Here's how the part is built. I have some questions about the finished solid (model axes, mm). Face numbers are marked on the shaded views. A direction names the side the tool comes from. Coordinates: 2 decimals unless noted, no trailing zeros. Loops run counter-clockwise (first coordinate to the right, second up) from the corner with the lowest first, then second, coordinate; pieces in that order, holes last.
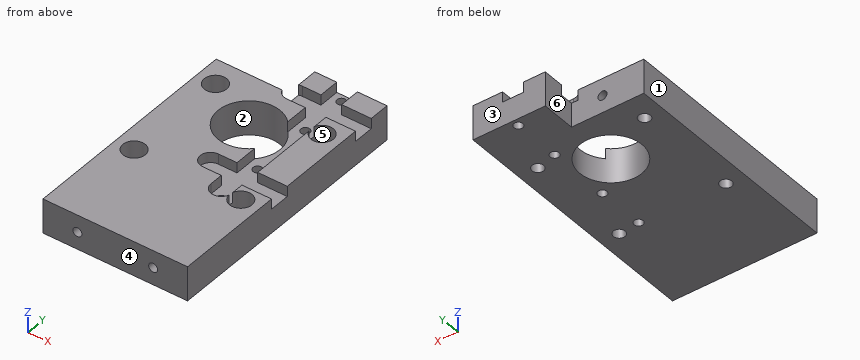
```python
from build123d import *

# Parameters (mm, degrees)
BOSS_EXTRUDE1_DEPTH                      = 10
CUT_EXTRUDE1_REACH                       = 89.407
SKETCH2_R                                = 9
CUT_EXTRUDE2_DEPTH                       = 3
CBORE_FOR_M3_PAN_HEAD_SCREW1_D           = 3.4
CBORE_FOR_M3_PAN_HEAD_SCREW1_CBORE_D     = 6.5
CBORE_FOR_M3_PAN_HEAD_SCREW1_CBORE_DEPTH = 6.5
M3X0_5_TAPPED_HOLE1_D                    = 2.6
M3X0_5_TAPPED_HOLE2_D                    = 2.6
M3X0_5_TAPPED_HOLE2_DEPTH                = 9
M3X0_5_TAPPED_HOLE2_TIP                  = 0.781118805
M3X0_5_TAPPED_HOLE3_D                    = 2.6
M3X0_5_TAPPED_HOLE3_DEPTH                = 9
M3X0_5_TAPPED_HOLE3_TIP                  = 0.781118805


with BuildPart() as part:
    # Sketch1 → Boss-Extrude1 (new body)
    with BuildSketch(Plane.XY):
        Polygon((0, 0), (42, 0), (42, 66), (42, 76), (21, 76), (21, 66), (0, 66), align=None)
    extrude(amount=BOSS_EXTRUDE1_DEPTH)

    # Sketch2 → Cut-Extrude1 (cut, up to next)
    with BuildSketch(Plane.XY.offset(10), mode=Mode.PRIVATE) as cut_extrude1_sk1:
        with Locations((21, 51)):
            Circle(SKETCH2_R)
    cut_extrude1_tool1 = extrude(cut_extrude1_sk1.sketch, amount=-CUT_EXTRUDE1_REACH, mode=Mode.PRIVATE) & part.part
    add(cut_extrude1_tool1.solids().sort_by_distance((21, 51, 10))[0], mode=Mode.SUBTRACT)

    # Sketch3 → Cut-Extrude2 (cut)
    with BuildSketch(Plane.XY.offset(10)):
        with BuildLine():
            Line((27.4, 32), (27.4, 28.1))
            ThreePointArc((27.4, 28.1), (30.4, 25.1), (33.4, 28.1))
            Line((33.4, 28.1), (33.4, 32))
            Line((33.4, 32), (42, 32))
            Line((42, 32), (42, 38))
            Line((42, 38), (33.4, 38))
            Line((33.4, 38), (33.4, 64))
            Line((33.4, 64), (42, 64))
            Line((42, 64), (42, 70))
            Line((42, 70), (33.4, 70))
            Line((33.4, 70), (33.4, 76))
            Line((33.4, 76), (27.4, 76))
            Line((27.4, 76), (27.4, 70))
            Line((27.4, 70), (22, 70))
            ThreePointArc((22, 70), (19, 67), (22, 64))
            Line((22, 64), (27.4, 64))
            Line((27.4, 64), (27.4, 38))
            Line((27.4, 38), (22, 38))
            ThreePointArc((22, 38), (19, 35), (22, 32))
            Line((22, 32), (27.4, 32))
        make_face()
    extrude(amount=-CUT_EXTRUDE2_DEPTH, mode=Mode.SUBTRACT)

    # CBORE for M3 Pan Head Screw1 (through all)
    with Locations(Plane.XY.offset(10)):
        with Locations((5.5, 58.5), (36.5, 58.5), (5.5, 27.5), (36.5, 27.5)):
            CounterBoreHole(CBORE_FOR_M3_PAN_HEAD_SCREW1_D / 2, CBORE_FOR_M3_PAN_HEAD_SCREW1_CBORE_D / 2, CBORE_FOR_M3_PAN_HEAD_SCREW1_CBORE_DEPTH)

    # M3x0.5 Tapped Hole1 (through all)
    with Locations(Plane.XY.offset(7)):
        with Locations((30.4, 73.9), (30.4, 60.1), (30.4, 41.9), (30.4, 28.1)):
            Hole(M3X0_5_TAPPED_HOLE1_D / 2)

    # M3x0.5 Tapped Hole2
    with Locations(Plane(origin=(0, 0, 0), x_dir=(-1, 0, 0), z_dir=(0, -1, 0))):
        with Locations((-10, -5), (-32, -5)):
            Hole(M3X0_5_TAPPED_HOLE2_D / 2, depth=M3X0_5_TAPPED_HOLE2_DEPTH)
            with Locations((0, 0, -(M3X0_5_TAPPED_HOLE2_DEPTH + M3X0_5_TAPPED_HOLE2_TIP / 2))):  # 118° drill point
                Cone(0, M3X0_5_TAPPED_HOLE2_D / 2, M3X0_5_TAPPED_HOLE2_TIP, mode=Mode.SUBTRACT)

    # M3x0.5 Tapped Hole3
    with Locations(Plane(origin=(0, 66, 0), x_dir=(1, 0, 0), z_dir=(0, 1, 0))):
        with Locations((12, -5)):
            Hole(M3X0_5_TAPPED_HOLE3_D / 2, depth=M3X0_5_TAPPED_HOLE3_DEPTH)
            with Locations((0, 0, -(M3X0_5_TAPPED_HOLE3_DEPTH + M3X0_5_TAPPED_HOLE3_TIP / 2))):  # 118° drill point
                Cone(0, M3X0_5_TAPPED_HOLE3_D / 2, M3X0_5_TAPPED_HOLE3_TIP, mode=Mode.SUBTRACT)


solid = part.part
```
1. I want a section at B-B (x = 5.5). Please give me the cut outline in (y, z).
2. I want a section at D-D (y = 35). Please give me the cut outline in (x, z), then the cut area to 3 significant figures.
3. On a 3-axis mill with a long thin cutter (end or side, diameter ignored), from which of +Z, -Z, +X, -X, +Y, -Y can I reach the whole of each face in a straight line? I mean the marked faces 4, 5 and 6. Say none if no direction works.
4. We'd pull the mould along X, two halves only. Please class the marked faces 1, 2 and 3: +X half, -X half, draft (parallel to the pull), parting line (faces both ways), or undercut.
5. I want a section at C-C (z = 1.25). Give the number of separate pieces and of enclosed holes in the cut face, then the cut area to 3 significant figures.
6. For pin 1 (5 mm diameter, centred on x = 26, z = 1, fed in from -Y); pin 2 (5 mm diameter, centred on x = 36.5, y = 58.5, fed in from +Z); pin 3 (0.9 mm diameter, centred on y = 72, z = 9, fed in from -X); pin 4 (2 mm diameter, centred on x = 29.5, y = 42, fed in from +Z), each with a flat end and sliding along its axis, tell me the tip position at first contact or that it passes through.
7. I need wall thicknesses on line 1 along Y through (x, z) = (5.5, 7); line 2 along Y through (x, z) = (5.5, 2.7); line 3 along Y through (x, z) = (30.4, 4.5). Which ranges of each line are inside material? Lowest first, please.
8. I want a section at A-A (y = 73.9). Please give me the cut outline in (x, z), then the cut area to 3 significant figures.
Response values:
1. outline: (0, 0) - (25.8, 0) - (25.8, 3.5) - (24.25, 3.5) - (24.25, 10) - (0, 10) - close; (29.2, 0) - (56.8, 0) - (56.8, 3.5) - (55.25, 3.5) - (55.25, 10) - (30.75, 10) - (30.75, 3.5) - (29.2, 3.5) - close; (60.2, 0) - (66, 0) - (66, 10) - (61.75, 10) - (61.75, 3.5) - (60.2, 3.5) - close
2. outline: (0, 0) - (42, 0) - (42, 7) - (19, 7) - (19, 10) - (0, 10) - close
2. area: 351 mm2
3. face 4: +Z, -Z, +X, -X, -Y
3. face 5: +Z
3. face 6: +Z, -Z, -X, +Y
4. face 1: -X half
4. face 2: undercut
4. face 3: draft
5. separate pieces: 1
5. enclosed holes: 9
5. area: 2,670 mm2
6. pin 1: stops at y = 0
6. pin 2: stops at z = 3.5
6. pin 3: stops at x = 21
6. pin 4: stops at z = 7
7. line 1: y = 0 to 24.25, 30.75 to 55.25, 61.75 to 66
7. line 2: y = 0 to 25.8, 29.2 to 56.8, 60.2 to 66
7. line 3: y = 0 to 26.8, 29.4 to 40.6, 43.2 to 58.8, 61.4 to 72.6, 75.2 to 76
8. outline: (21, 0) - (29.1, 0) - (29.1, 7) - (27.4, 7) - (27.4, 10) - (21, 10) - close; (31.7, 0) - (42, 0) - (42, 10) - (33.4, 10) - (33.4, 7) - (31.7, 7) - close
8. area: 174 mm2
